Source: CAD feature listing. Evaluate the final solid. Frame: model axes, mm. A direction names the side the tool comes from. Round coordinates to 2 decimals unless told otherwise and drop trailing zeros. Order: outer loops, then holes, each group sorted by start corner. A loop starts at its lowest first (then second) coordinate and runs counter-clockwise, first axis right, second up. Notation, with made-up numbers: (-3, 38.5) - (31, 38.5) arc R8 cw to (31, 50.5) - close; hole circle Ø2 at (74, 17.5). An arc over 180 degrees is marked (long way). Return JSON: item names as keys, results as strings. Group by question number.
1) Section C-C, the plane x = 2.5. Return loops of the section in (y, z) (3 decimals), plus the area to 3 significant figures.
2) Contact query for flat-ended pins moving along their axis: P1, Ø10, axis at x = 12, z = -7, coming from the -Y side; P2, Ø10, axis at y = 10.5, z = 10.5, coming from the +X side; P3, Ø7, axis at x = 13.5, z = -29.5, coming from the -Y side; P4, Ø2, axis at x = 12.5, z = -9.5, coming from the -Y side. Output: stop coordinate, or through.
3) Section A-A, the plane x = 14. Give the number of separate pieces and of enclosed holes in the cut face, plus the area to 3 significant figures.
4) Section B-B, the plane z = -1. Return loops of the section in (x, y) (3 decimals).
5) Mould query, pull axis Z, two halves, no side actions, for faces 5 (the flat face through (17.78, 24, -29)), 6 (the flat face through (5.6, 12.4, 13.1)), 7 (the cylindrical face through (6, 4, -1)). Classes: pulls with the +Z half, pulls with the -Z half, needs draft (parallel to the pull), parting line crosses it, or undercut.
6) Section D-D, the plane y = 6.35. Return loops of the section in (x, z).
7) Ray query, line 1 (Y direction, x = 15.75, z = -31.75) (3 decimals); line 2 (Z direction, x = 16.75, y = 25.4); line 3 (Z direction, x = 13.25, y = 17). Return the intervals inside material, ascending. Write a range as from..to.
8) Access query for faces 1 (the flat face through (19, -25, 19.05)), 2 (the flat face through (15, 15.875, -28)), 3 (the cylindrical face through (18.638, -26.007, 29.824)), 4 (the flat face through (19, -22.225, 29)). Directions: +Z, -Z, +X, -X, +Y, -Y. A direction counts if a zero-diameter tool reaches every point of the face in a straight line with its end or side. Return the directions, or none.
```python
from build123d import *

# Parameters (mm, degrees)
SKETCH1_W                   = 76.2
SKETCH1_H                   = 63.5
BOSS_EXTRUDE1_DEPTH         = 25.4
SKETCH2_W                   = 38.1
SKETCH2_H                   = 63.5
CUT_EXTRUDE1_DEPTH          = 13.97
F_1_4_20_TAPPED_HOLE1_D     = 5.1054
F_1_4_20_TAPPED_HOLE1_DEPTH = 19.05
F_1_4_20_TAPPED_HOLE1_TIP   = 1.533816902
LPATTERN1_COUNT             = 2
LPATTERN1_PITCH             = 50.8
LPATTERN1_COUNT_DIR2        = 2
LPATTERN1_PITCH_DIR2        = 63.5
SKETCH7_W                   = 76.2
SKETCH7_H                   = 38.1
CUT_EXTRUDE2_DEPTH          = 13.97
SKETCH8_OUTSIDE_W           = 98.678
SKETCH8_OUTSIDE_H           = 85.978
CUT_EXTRUDE3_DEPTH          = 56.72102386
SKETCH9_W                   = 7.62
SKETCH9_H                   = 15.875
CUT_EXTRUDE4_DEPTH          = 87.36933773


with BuildPart() as part:
    # Sketch1 → Boss-Extrude1 (new body)
    with BuildSketch(Plane(origin=(0, 0, 0), x_dir=(0, 0, -1), z_dir=(1, 0, 0))):
        Rectangle(SKETCH1_W, SKETCH1_H)
    extrude(amount=BOSS_EXTRUDE1_DEPTH)

    # Sketch2 → Cut-Extrude1 (cut)
    with BuildSketch(Plane(origin=(25.4, 0, 0), x_dir=(0, 0, -1), z_dir=(1, 0, 0))):
        Rectangle(SKETCH2_W, SKETCH2_H)
    extrude(amount=-CUT_EXTRUDE1_DEPTH, mode=Mode.SUBTRACT)

    # Sketch5 → #10-32 Tapped Hole1 (revolve, cut)
    with BuildSketch(Plane(origin=(25.4, 25.4, 31.75), x_dir=(0, 0, -1), z_dir=(0, 1, 0))):
        Polygon((0, 0), (0, 14.929317848), (2.0193, 13.716), (2.0193, 0), align=None)
    f_10_32_tapped_hole1 = revolve(axis=Axis((31.75, 25.4, 31.75), (-1, 0, 0)), mode=Mode.SUBTRACT)

    # 1/4-20 Tapped Hole1
    with Locations(Plane(origin=(11.43, 0, 0), x_dir=(0, 0, -1), z_dir=(1, 0, 0))):
        with Locations((0, 6.35)):
            Hole(F_1_4_20_TAPPED_HOLE1_D / 2, depth=F_1_4_20_TAPPED_HOLE1_DEPTH)
            with Locations((0, 0, -(F_1_4_20_TAPPED_HOLE1_DEPTH + F_1_4_20_TAPPED_HOLE1_TIP / 2))):  # 118° drill point
                Cone(0, F_1_4_20_TAPPED_HOLE1_D / 2, F_1_4_20_TAPPED_HOLE1_TIP, mode=Mode.SUBTRACT)

    # LPattern1: 10-32 Tapped Hole1 2 × 2
    with Locations(*[(0, -i * LPATTERN1_PITCH, -j * LPATTERN1_PITCH_DIR2) for i in range(LPATTERN1_COUNT) for j in range(LPATTERN1_COUNT_DIR2) if (i, j) != (0, 0)]):
        add(f_10_32_tapped_hole1, mode=Mode.SUBTRACT)

    # Sketch7 → Cut-Extrude2 (cut)
    with BuildSketch(Plane(origin=(25.4, 0, 0), x_dir=(0, 0, -1), z_dir=(1, 0, 0))):
        with Locations((0, -3.175)):
            Rectangle(SKETCH7_W, SKETCH7_H)
    extrude(amount=-CUT_EXTRUDE2_DEPTH, mode=Mode.SUBTRACT)

    # Sketch8 outside → Cut-Extrude3 (cut, through all)
    with BuildSketch(Plane.ZY):
        Rectangle(SKETCH8_OUTSIDE_W, SKETCH8_OUTSIDE_H)
        Polygon((-38.1, 15.875), (25.4, -31.75), (38.1, -31.75), (39.3192, -7.2644), (-12.7, 31.75), (-38.1, 31.75), align=None, mode=Mode.SUBTRACT)
    extrude(amount=-CUT_EXTRUDE3_DEPTH, mode=Mode.SUBTRACT)

    # Sketch9 → Cut-Extrude4 (cut, through all)
    with BuildSketch(Plane(origin=(0, 0, -38.1), x_dir=(-1, 0, 0), z_dir=(0, 0, -1))):
        with Locations((-21.59, 23.8125)):
            Rectangle(SKETCH9_W, SKETCH9_H)
    extrude(amount=-CUT_EXTRUDE4_DEPTH, mode=Mode.SUBTRACT)


solid = part.part
```
Geometry check:
{
 "1": {"outline": "(-31.75, 25.4) - (15.875, -38.1) - (31.75, -38.1) - (31.75, -12.7) - (-6.35, 38.1) - (-31.75, 38.1) - close; hole circle Ø5.105 at (6.35, 0)", "area": "2,340 mm2"},
 "2": {"P1": "y = -11.18", "P2": "x = 11.43", "P3": "y = 7.31", "P4": "through"},
 "3": {"separate pieces": "2", "enclosed holes": "2", "area": "443 mm2"},
 "4": {"outline": "(0, -11.95) - (11.43, -11.95) - (11.43, 4.001) - (0, 4.001) - close; (0, 8.699) - (11.43, 8.699) - (11.43, 22.975) - (0, 22.975) - close"},
 "5": {"face 5": "needs draft", "face 6": "pulls with the +Z half", "face 7": "undercut"},
 "6": {"outline": "(0, -25.4) - (11.43, -25.4) - (11.43, -2.55) - (0, -2.55) - close; (0, 2.55) - (11.43, 2.55) - (11.43, 21.17) - (0, 21.17) - close"},
 "7": {"line 1": "15.875..23.381, 27.419..31.75", "line 2": "-38.1..-33.77, -29.73..-19.05", "line 3": "-38.1..-19.05"},
 "8": {"face 1": "-Z, +X, +Y, -Y", "face 2": "+Z, -Z, +X, -Y", "face 3": "+X", "face 4": "+Z, -Z, +X, +Y"}
}
